The listing builds one solid part. Answer for the finished solid, in the listing's coordinates (mm). A direction names the side the tool comes from. Give positions to 0.01 mm unless a question says otherwise; leave off trailing zeros. Order: outer loops, then holes, each group sorted by start corner. A loop starts at its lowest first (then second) coordinate and runs counter-clockwise, first axis right, second up. Notation, with made-up numbers: (59.5, -7.5) - (112.5, -7.5) arc R13 cw to (112.5, 6.5) - close; hole circle Ø4 at (41.5, 60). An arc over 180 degrees is marked (long way). Answer as a JSON object with one key per item and string values. Group by question number.
Q1. A cutting plane is placed at A-A, the plane z = 0.5. Give the vertices of the cut face in (x, y).
Q2. Consider line 1 (Z direction, x = 0, y = 0.75); line 2 (Z direction, x = -1.65, y = 18); line 3 (Z direction, x = 0.45, y = 25.5). Determine where each line is inside the solid, lowest interval first.
Q3. A cutting plane is placed at D-D, the plane z = -3.75. Give the vertices of the cut face in (x, y), and give its area (3 significant figures).
Q4. Given pin 1 (6 mm diameter, centred on y = 25, z = -3, fed in from +X); pin 2 (1 mm diameter, centred on x = 1, y = 23, fed in from +Z); pin 3 (1 mm diameter, centred on x = 0, z = -2.5, fed in from -Y), each flat-ended and moving along its own axis, determine where each tip first touches the part or whether it passes through.
Q5. A cutting plane is placed at B-B, the plane x = -1.3. Give the vertices of the cut face in (y, z).
Q6. The mould has two halves that part along X. Classify faces 1 (the face through (0, 0, 0)), 2 (the face through (0.221, 0.74, -4.186)), 3 (the face through (2.5, 7, 0)): released by +X, released by -X, zero draft, split by the parting line, or undercut.
Q7. For faces 4 (the face through (0, 1.5, 3)), 5 (the face through (0.035, 20.414, 4.045)), determine the directions among +Z, -Z, +X, -X, +Y, -Y from which every point of the face is accessible in a straight line to the end or side of a thin tool.
Q8. A cutting plane is placed at C-C, the plane y = 20. Give the vertices of the cut face in (x, z).
Autodesk Inventor part; units mm, degrees
ref_plane "YZ Plane" through (0, 0, 0) normal (1, 0, 0) x (0, 1, 0)
ref_plane "XZ Plane" through (0, 0, 0) normal (0, 1, 0) x (-1, 0, 0)
ref_plane "XY Plane" through (0, 0, 0) normal (0, 0, 1) x (1, 0, 0)
sketch "草圖1" plane through (0, 0, 0) normal (0, 1, 0) x (-1, 0, 0)
  line L0 (2.5, 5) -> (-2.5, 5)
  line L1 (-2.5, 5) -> (-2.5, -5)
  line L2 (-2.5, -5) -> (2.5, -5)
  line L3 (2.5, -5) -> (2.5, 5)
  circle A0 centre (0, 2.5) radius 1.7
  point P0 (0, 0)
  point P1 (0, -5)
  point P2 (2.5, 0)
  dimension "d0" = 5
  dimension "d1" = 10
  dimension "d2" = 3.4
  dimension "d3" = 2.5
  dimension "d4" = 2.5
extrude "擠出1" add sketch "草圖1" along normal blind 15 contours L3 L2 L1 L0 | A0
extrude "擠出2" cut sketch "草圖1" along normal blind 1.5 contours A0
pattern_linear "矩形陣列1" count 2 spacing 5 along (0, 0, -1) of "擠出2"
sketch "草圖3" plane through (0, 15, 0) normal (0, 1, 0) x (1, 0, 0)
  line L0 (2.5, -5) -> (2.5, 5)
  line L1 (2.5, 5) -> (-2.5, 5)
  line L2 (-2.5, 5) -> (-2.5, -5)
  line L3 (-2.5, -5) -> (2.5, -5)
  point P0 (0, 0)
extrude "擠出4" add sketch "草圖3" along normal blind 20 draft -10
properties part number "110033226_ipt_40_背流拱橋裝飾"
Reply:
{
 "1": {"outline": "(-2.5, 0) - (2.5, 0) - (2.5, 15) - (0, 29.18) - (-2.5, 15) - close"},
 "2": {"line 1": "z = -5 to -4.2, -0.8 to 0.8, 4.2 to 5", "line 2": "z = -4.47 to 4.47", "line 3": "z = -3.15 to 3.15"},
 "3": {"outline": "(-2.5, 0) - (-1.15, 0) - (-1.15, 1.5) - (1.15, 1.5) - (1.15, 0) - (2.5, 0) - (2.5, 15) - (1.25, 22.09) - (-1.25, 22.09) - (-2.5, 15) - close", "area": "98.1 mm^2"},
 "4": {"pin 1": "stops at x = 1.27", "pin 2": "stops at z = 3.68", "pin 3": "stops at y = 1.5"},
 "5": {"outline": "(0, -5) - (15, -5) - (21.81, -3.8) - (21.81, 3.8) - (15, 5) - (0, 5) - (0, 3.6) - (1.5, 3.6) - (1.5, 1.4) - (0, 1.4) - (0, -1.4) - (1.5, -1.4) - (1.5, -3.6) - (0, -3.6) - close"},
 "6": {"face 1": "zero draft", "face 2": "undercut", "face 3": "released by +X"},
 "7": {"face 4": "-Y", "face 5": "+Z, +X, -X, +Y"},
 "8": {"outline": "(-1.62, -4.12) - (1.62, -4.12) - (1.62, 4.12) - (-1.62, 4.12) - close"}
}
